Answer from the drawing. Dimensions are ordinates in mm from the lowest x, y and z of the part. A direction names the side the tool comes from. Coordinates: 2 decimals unless noted, no trailing zeros. Write each loop counter-clockwise with the first axis right and the second up, starting at its lowest first coordinate (ties: lowest second). Pieces come first, ordered by that corner, then holes.
1) Find the intervals of material crossed by line 1 (Z direction, x = 6, y = 56); line 2 (Y direction, x = 11, z = 9.5); line 3 (Y direction, x = 5, z = 5.5), in increasing order.
2) Which of the six approach directions +Z, -Z, +X, -X, +Y, -Y give full straight-line access (tool end or side, diameter ignored) to the marked faces 1, 2 and 3?
3) Each of these flat-tipped pins is pushed along its axis until it touches: pin 1 Ø3.5 at (y, z) = (56, 6.35) entering from +X; pin 2 Ø2 at (x, z) = (12, 7.5) entering from +Y; pin 3 Ø3 at (x, y) = (10.5, 29) entering from -Z. Where does it stop, or does it pass through?
4) The part is cut by section C-C (x = 5). Determine the outline of the cut face in (y, z).
5) The part is cut by section D-D (z = 2.5). Determine the outline of the cut face in (x, y).
6) The part is cut by section A-A (z = 6.35). Determine the outline of the cut face in (x, y).
7) The part is cut by section B-B (y = 56). Determine the outline of the cut face in (x, z).
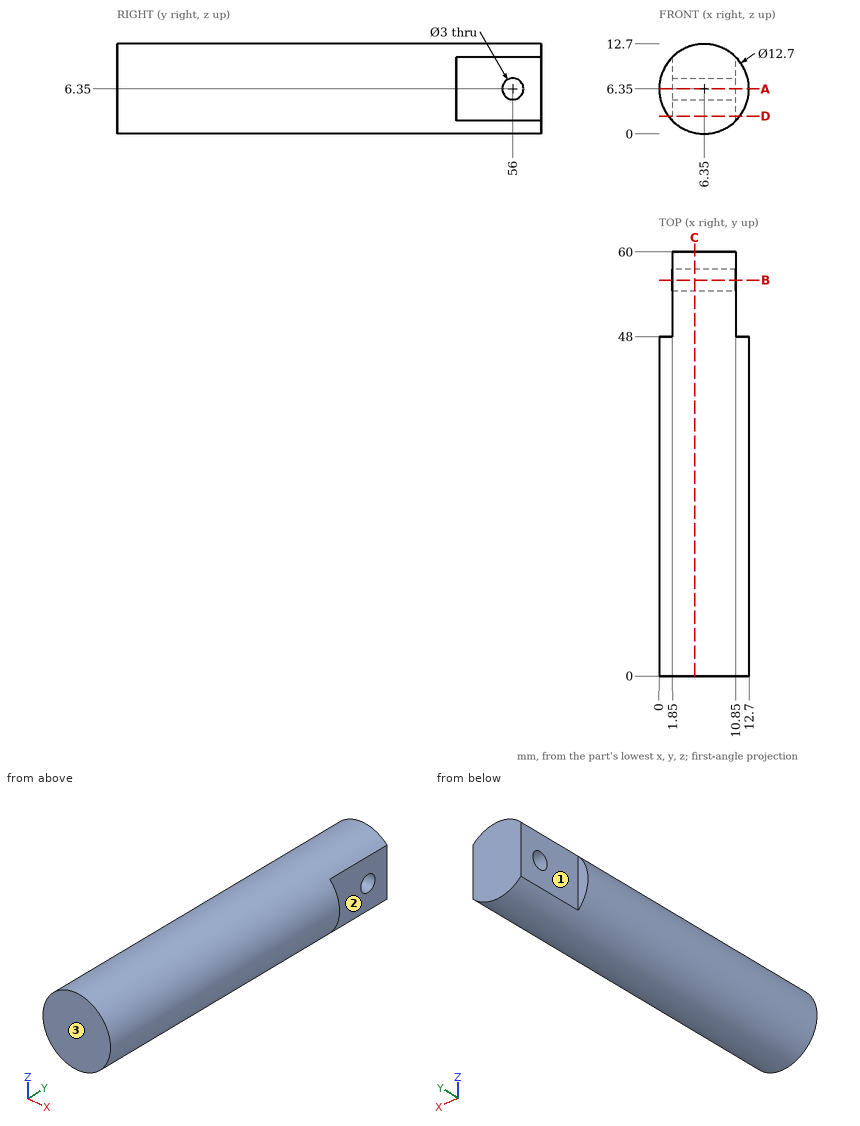
Reported:
1. line 1: z = 0.01 to 4.85, 7.85 to 12.69
1. line 2: y = 0 to 48
1. line 3: y = 0 to 54.76, 57.24 to 60
2. face 1: +Z, -Z, -X, +Y
2. face 2: +Z, -Z, +X, +Y
2. face 3: +Z, -Z, +X, -X, -Y
3. pin 1: stops at x = 10.85
3. pin 2: stops at y = 48
3. pin 3: stops at z = 0.58
4. outline: (0, 0.15) - (60, 0.15) - (60, 12.55) - (0, 12.55) - close; hole circle Ø3 at (56, 6.35)
5. outline: (1.3, 0) - (11.4, 0) - (11.4, 48) - (10.85, 48) - (10.85, 60) - (1.85, 60) - (1.85, 48) - (1.3, 48) - close
6. outline: (0, 0) - (12.7, 0) - (12.7, 48) - (10.85, 48) - (10.85, 54.5) - (1.85, 54.5) - (1.85, 48) - (0, 48) - close; (1.85, 57.5) - (10.85, 57.5) - (10.85, 60) - (1.85, 60) - close
7. outline: (1.85, 1.87) arc R6.35 ccw to (10.85, 1.87) - (10.85, 4.85) - (1.85, 4.85) - close; (1.85, 7.85) - (10.85, 7.85) - (10.85, 10.83) arc R6.35 ccw to (1.85, 10.83) - close
